from build123d import *

# Parameters (mm, degrees)
BOSS_EXTRUDE1_DEPTH = 4.75
SKETCH2_R           = 2.25
CUT_EXTRUDE1_DEPTH  = 10
FILLET1_R           = 4


with BuildPart() as part:
    # Sketch1 → Boss-Extrude1 (new body, symmetric)
    with BuildSketch(Plane(origin=(0, 0, 0), x_dir=(1, 0, 0), z_dir=(0, 1, 0))):
        with BuildLine():
            Line((0, -3.5), (-16.5, -3.5))
            Line((-16.5, -3.5), (-16.5, -4.5))
            Line((-16.5, -4.5), (0, -4.5))
            ThreePointArc((0, -4.5), (3.354101966, 3), (-4.472135955, 0.5))
            Line((-4.472135955, 0.5), (-16.5, 0.5))
            Line((-16.5, 0.5), (-16.5, -0.5))
            Line((-16.5, -0.5), (-3.464101615, -0.5))
            ThreePointArc((-3.464101615, -0.5), (2.291287847, 2.645751311), (0, -3.5))
        make_face()
    extrude(amount=BOSS_EXTRUDE1_DEPTH, both=True)

    # Sketch2 → Cut-Extrude1 (cut, through all)
    with BuildSketch(Plane.XY.offset(4.5)):
        with Locations((-12, 0)):
            Circle(SKETCH2_R)
    extrude(amount=-CUT_EXTRUDE1_DEPTH, mode=Mode.SUBTRACT)

    # Fillet1
    fillet1_edges = [part.edges().sort_by_distance(p)[0] for p in [
        (-16.5, 4.75, 4),
        (-16.5, 4.75, 0),
        (-16.5, -4.75, 0),
        (-16.5, -4.75, 4),
    ]]
    fillet(fillet1_edges, radius=FILLET1_R)


solid = part.part
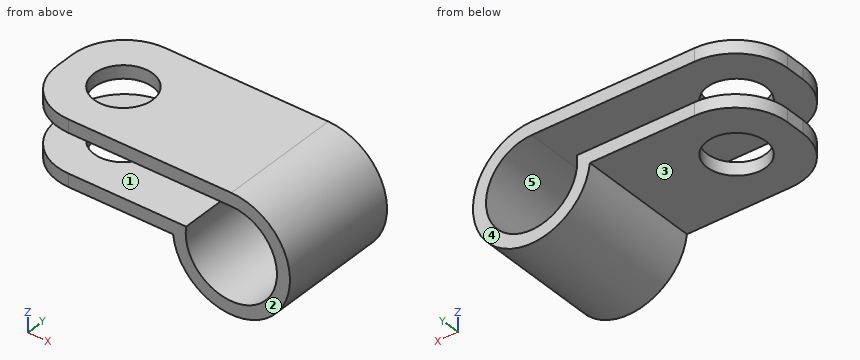
Verification items for the finished model (mm, model axes). Face numbers are marked on the shaded views. A direction names the side the tool comes from. Coordinates: 2 decimals unless noted, no trailing zeros. Order: outer loops, then holes, each group sorted by start corner. A loop starts at its lowest first (then second) coordinate and runs counter-clockwise, first axis right, second up.
1. Sectioned sample at B-B, the plane x = -12. Record the cut outline in (y, z).
Results found:
outline: (-4.75, -0.5) - (-2.25, -0.5) - (-2.25, 0.5) - (-4.75, 0.5) - close; (-4.75, 3.5) - (-2.25, 3.5) - (-2.25, 4.5) - (-4.75, 4.5) - close; (2.25, -0.5) - (4.75, -0.5) - (4.75, 0.5) - (2.25, 0.5) - close; (2.25, 3.5) - (4.75, 3.5) - (4.75, 4.5) - (2.25, 4.5) - close
2. Set-up check for the marked faces 1 and 2: record each of +Z, -Z, +X, -X, +Y, -Y from which the full face is reachable in a straight line by a thin tool's end or side.
Results found:
face 1: -X, +Y, -Y
face 2: +Z, -Z, +X, -X, -Y
3. Sectioned sample at A-A, the plane z = 0. Record the cut outline in (x, y).
Results found:
outline: (-16.5, -0.75) arc R4 ccw to (-12.5, -4.75) - (-3.5, -4.75) - (-3.5, 4.75) - (-12.5, 4.75) arc R4 ccw to (-16.5, 0.75) - close; (3.5, -4.75) - (4.5, -4.75) - (4.5, 4.75) - (3.5, 4.75) - close; hole circle Ø4.5 at (-12, 0)
4. Sectioned sample at C-C, the plane y = 0. Record the cut outline in (x, z), and give its area (3 significant figures).
Results found:
outline: (-16.5, -0.5) - (-14.25, -0.5) - (-14.25, 0.5) - (-16.5, 0.5) - close; (-16.5, 3.5) - (-14.25, 3.5) - (-14.25, 4.5) - (-16.5, 4.5) - close; (-9.75, -0.5) - (-4.47, -0.5) arc R4.5 ccw (long way) to (0, 4.5) - (-9.75, 4.5) - (-9.75, 3.5) - (0, 3.5) arc R3.5 cw (long way) to (-3.46, 0.5) - (-9.75, 0.5) - close
area: 38.9 mm2
5. Go/stop test with flat-tipped pins: pin 1 Ø2 at (y, z) = (-3, 1) entering from -X; pin 2 Ø1 at (x, y) = (-11, 2) entering from -Z. Record where each tip stops, or that it passes through.
Results found:
pin 1: stops at x = -16.25
pin 2: stops at z = -0.5
6. Release check for a two-part mould opening along Z. For the marked faces 3, 4 and 5 record: +Z half, -Z half, draft (parallel to the pull), parting line (faces both ways), or undercut.
Results found:
face 3: -Z half
face 4: draft
face 5: undercut
7. Scan lines: line 1 (Y direction, x = -12, z = 0.35); line 2 (Z direction, x = -12, y = 2.5); line 3 (Z direction, x = -0.5, y = 2.75). Record each from-to range of solid material in increasing order.
Results found:
line 1: y = -4.75 to -2.25, 2.25 to 4.75
line 2: z = -0.5 to 0.5, 3.5 to 4.5
line 3: z = -4.47 to -3.46, 3.5 to 4.5
8. Sectioned sample at D-D, the plane x = -5. Record the cut outline in (y, z).
Results found:
outline: (-4.75, -0.5) - (4.75, -0.5) - (4.75, 0.5) - (-4.75, 0.5) - close; (-4.75, 3.5) - (4.75, 3.5) - (4.75, 4.5) - (-4.75, 4.5) - close
